Geometry check sheet. Reference: drawing and pictorial views, mm from the part's lowest x, y, z. Give positions to 0.01 mm unless a question says otherwise; leave off trailing zeros. Loops run counter-clockwise (first coordinate to the right, second up) from the corner with the lowest first, then second, coordinate; pieces in that order, holes last. Notation, with made-up numbers: M 40.5,-27.75 L 54.5,-27.75 A17 cw 54.5,-11.75 Z; hole C 24.5,18.25 d3. An arc over 180 degrees is marked long. Use CSV: the item, a comma, the result in double quotes.
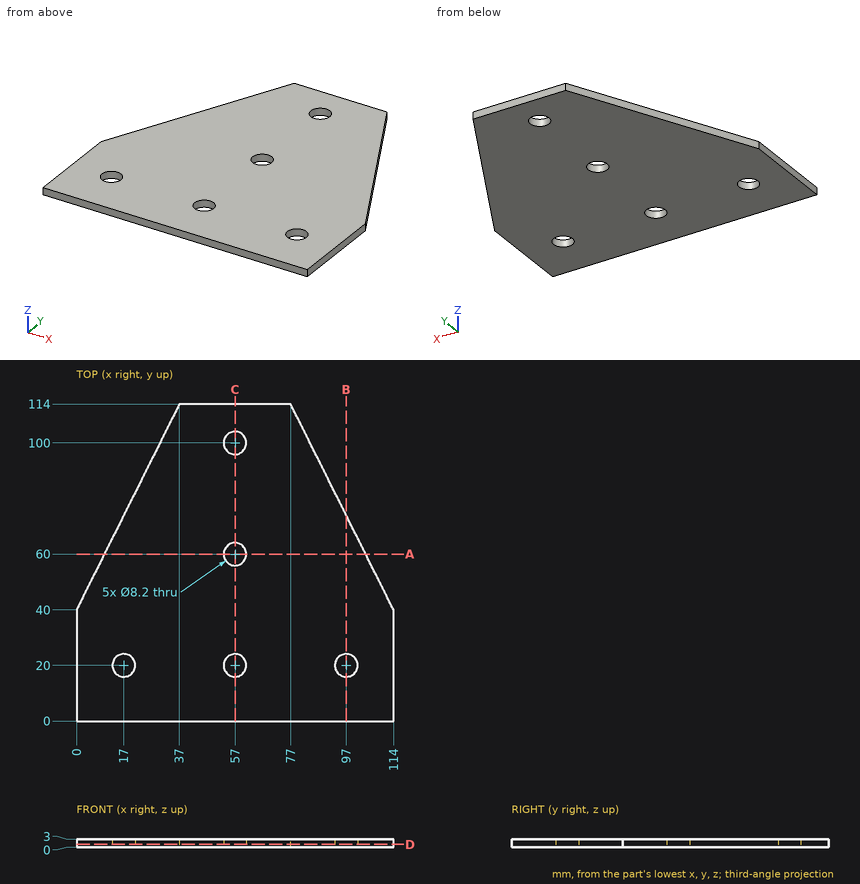
(1) Section check B-B on x = 97. Record the cut outline in (y, z).
Calculated:
outline,"M 0,0 L 15.9,0 L 15.9,3 L 0,3 Z; M 24.1,0 L 74,0 L 74,3 L 24.1,3 Z"
(2) Section check C-C on x = 57. Record the cut outline in (y, z).
Calculated:
outline,"M 0,0 L 15.9,0 L 15.9,3 L 0,3 Z; M 24.1,0 L 55.9,0 L 55.9,3 L 24.1,3 Z; M 64.1,0 L 95.9,0 L 95.9,3 L 64.1,3 Z; M 104.1,0 L 114,0 L 114,3 L 104.1,3 Z"
(3) Section check A-A on y = 60. Record the cut outline in (x, z), plus the area to 3 significant figures.
Calculated:
outline,"M 10,0 L 52.9,0 L 52.9,3 L 10,3 Z; M 61.1,0 L 104,0 L 104,3 L 61.1,3 Z"
area,"257 mm²"
(4) Scan lines: L1, parallel to Y at x = 57, z = 0.85; L2, parallel to X at y = 21.5, z = 2.55; L3, parallel to X at y = 98, z = 1.35. Record each from-to range of solid material in increasing order. Write a range as from..to.
Calculated:
L1,"y = 0..15.9, 24.1..55.9, 64.1..95.9, 104.1..114"
L2,"x = 0..13.18, 20.82..53.18, 60.82..93.18, 100.82..114"
L3,"x = 29..53.42, 60.58..85"
(5) Section check D-D on z = 1.05. Record the cut outline in (x, y).
Calculated:
outline,"M 0,0 L 114,0 L 114,40 L 77,114 L 37,114 L 0,40 Z; hole C 17,20 d8.2; hole C 57,20 d8.2; hole C 57,60 d8.2; hole C 57,100 d8.2; hole C 97,20 d8.2"
